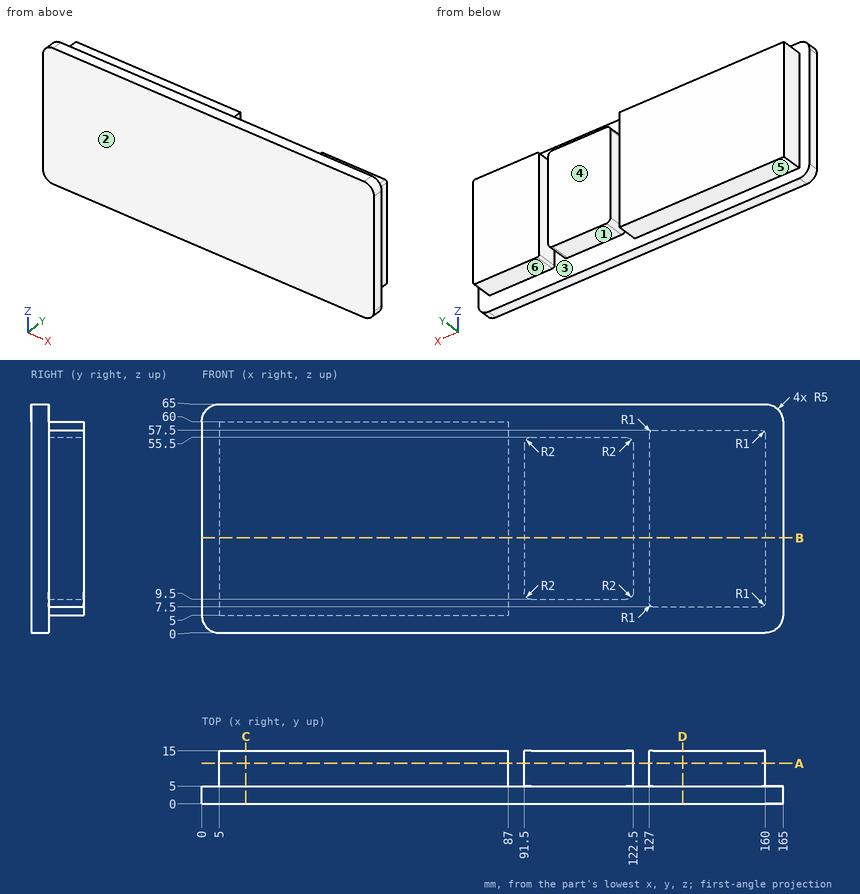
Answer from the drawing. Dimensions are ordinates in mm from the lowest x, y and z of the part. A direction names the side the tool comes from. Coordinates: 2 decimals unless noted, no trailing zeros. Write each loop counter-clockwise with the first axis right and the second up, starting at its lowest first coordinate (ties: lowest second). Pieces come first, ordered by that corner, then holes. Notation, with made-up numbers: M 22,33.25 L 29,33.25 A26 cw 29,68.25 Z; hole C 75.25,49 d11. An arc over 180 degrees is marked long. Use one line per item in the form item = value. Start each with the question number.
1. The part is cut by section A-A (y = 11.5). Give the vertices of the cut face in (x, z), plus the area to 3 significant figures.
2. Each of these flat-tipped pins is pushed along its axis until it touches: P1, Ø8, axis at x = 56, y = 11.5, coming from the +Z side; P2, Ø5, axis at y = 11, z = 30.5, coming from the +X side; P3, Ø3, axis at x = 111, y = 9.5, coming from the -Z side. Where does it stop, or does it pass through?
3. The part is cut by section C-C (x = 12.5). Give the vertices of the cut face in (y, z).
4. A tool of negligible diameter and unlimited length cuts with its end or side. For the marked faces 4, 5 and 6, from which of +Z, -Z, +X, -X, +Y, -Y can it reach the whole face along a straight path? Write none if from no direction.
5. The mould has two halves that part along X. Classify the marked faces 1, 2 and 3: released by +X, released by -X, zero draft, split by the parting line, or undercut.
6. The part is cut by section B-B (z = 27). Give the vertices of the cut face in (x, y).
7. Straight lines are drawn through the part: probe 1 along X at (y, z) = (7.75, 40); probe 2 along Z at (x, y) = (156, 13.25); probe 3 along Z at (x, y) = (41, 5.5). For each, find the intervals that lie inside material, in ascending order. Write a range as from..to.
8. The part is cut by section D-D (x = 136.5). Give the vertices of the cut face in (y, z), plus the area to 3 significant figures.
Evaluation:
q1.outline = M 5,5 L 87,5 L 87,60 L 5,60 Z; M 91.5,11.5 A2 ccw 93.5,9.5 L 120.5,9.5 A2 ccw 122.5,11.5 L 122.5,53.5 A2 ccw 120.5,55.5 L 93.5,55.5 A2 ccw 91.5,53.5 Z; M 127,8.5 A1 ccw 128,7.5 L 159,7.5 A1 ccw 160,8.5 L 160,56.5 A1 ccw 159,57.5 L 128,57.5 A1 ccw 127,56.5 Z
q1.area = 7,580 mm^2
q2.P1 = 60
q2.P2 = 160
q2.P3 = 9.5
q3.outline = M 0,0 L 5,0 L 5,5 L 15,5 L 15,60 L 5,60 L 5,65 L 0,65 Z
q4.face_4 = +Z, -Z, +X, -X, +Y
q4.face_5 = -Z, +X, -X, +Y
q4.face_6 = -Z, +X, +Y
q5.face_1 = undercut
q5.face_2 = zero draft
q5.face_3 = undercut
q6.outline = M 0,0 L 165,0 L 165,5 L 160,5 L 160,15 L 127,15 L 127,5 L 122.5,5 L 122.5,15 L 91.5,15 L 91.5,5 L 87,5 L 87,15 L 5,15 L 5,5 L 0,5 Z
q7.probe_1 = 5..87, 91.5..122.5, 127..160
q7.probe_2 = 7.5..57.5
q7.probe_3 = 5..60
q8.outline = M 0,0 L 5,0 L 5,7.5 L 15,7.5 L 15,57.5 L 5,57.5 L 5,65 L 0,65 Z
q8.area = 825 mm^2
